Geometry: final body of the model. Coordinates: model frame, mm. Give positions to 0.01 mm unless a question says otherwise; leave off trailing zeros. Loops run counter-clockwise (first coordinate to the right, second up) from the corner with the lowest first, then second, coordinate; pieces in that order, holes last.
Autodesk Inventor part; units mm, degrees
ref_plane "YZ Plane" through (0, 0, 0) normal (1, 0, 0) x (0, 1, 0)
ref_plane "XZ Plane" through (0, 0, 0) normal (0, 1, 0) x (-1, 0, 0)
ref_plane "XY Plane" through (0, 0, 0) normal (0, 0, 1) x (1, 0, 0)
sketch "スケッチ1" plane through (0, 0, 0) normal (0, 1, 0) x (-1, 0, 0)
  line L0 (-21.5, -21.5) -> (21.5, -21.5)
  line L1 (21.5, -21.5) -> (21.5, 21.5)
  line L2 (21.5, 21.5) -> (-21.5, 21.5)
  line L3 (-21.5, 21.5) -> (-21.5, -21.5)
  line L4 (-21.5, -21.5) -> (21.5, 21.5) construction
  line L5 (21.5, -21.5) -> (-21.5, 21.5) construction
  point P0 (0, 0)
  dimension "d0" = 43
  dimension "d1" = 43
extrude "押し出し1" add sketch "スケッチ1" along normal blind 18
chamfer "面取り1" distance 2 angle 45 1 edges at (21.5, 9, 21.5)
chamfer "面取り2" distance 2 angle 45 1 edges at (21.5, 9, -21.5)
chamfer "面取り3" distance 2 angle 45 1 edges at (-21.5, 9, 21.5)
chamfer "面取り4" distance 2 angle 45 1 edges at (-21.5, 9, -21.5)
sketch "スケッチ2" plane through (0, 0, 0) normal (0, 1, 0) x (-1, 0, 0)
  circle A0 centre (0, 0) radius 6
  dimension "d16" = 12
extrude "押し出し2" cut sketch "スケッチ2" along normal blind 18
properties part number "GearHead1"
Item 1: Pin query (flat end, axial travel): pin 1 (14 mm diameter, centred on x = 0, z = 0, fed in from -Y). Return the tip coordinate at first contact, or that it passes through.
Values follow:
pin 1: stops at y = 0
Item 2: Section query B-B on z = 0. Return loops of the section in (x, y).
Values follow:
outline: (-21.5, 0) - (-6, 0) - (-6, 18) - (-21.5, 18) - close; (6, 0) - (21.5, 0) - (21.5, 18) - (6, 18) - close
Item 3: Section query A-A on x = 0. Return loops of the section in (y, z), plus the area to 3 significant figures.
Values follow:
outline: (0, -21.5) - (18, -21.5) - (18, -6) - (0, -6) - close; (0, 6) - (18, 6) - (18, 21.5) - (0, 21.5) - close
area: 558 mm2
Item 4: Draft query along Z for faces 1 (the face through (6, 9, 0)), 2 (the face through (-21, 9, 20)), 3 (the face through (-20, 9, -21)), 4 (the face through (-4, 18, 5)). Return one class per face: +Z half, -Z half, draft (parallel to the pull), parting line (faces both ways), or undercut.
Values follow:
face 1: undercut
face 2: +Z half
face 3: -Z half
face 4: draft
Item 5: Ray query, probe 1 along Z at (x, y) = (0, 12.5); probe 2 along Z at (x, y) = (-1.5, 2); probe 3 along X at (y, z) = (16, 5.5). Return the intervals inside material, ascending.
Values follow:
probe 1: z = -21.5 to -6, 6 to 21.5
probe 2: z = -21.5 to -5.81, 5.81 to 21.5
probe 3: x = -21.5 to -2.4, 2.4 to 21.5
Item 6: Section query C-C on y = 11.75. Return loops of the section in (x, z).
Values follow:
outline: (-21.5, -19.5) - (-19.5, -21.5) - (19.5, -21.5) - (21.5, -19.5) - (21.5, 19.5) - (19.5, 21.5) - (-19.5, 21.5) - (-21.5, 19.5) - close; hole circle Ø12 at (0, 0)
